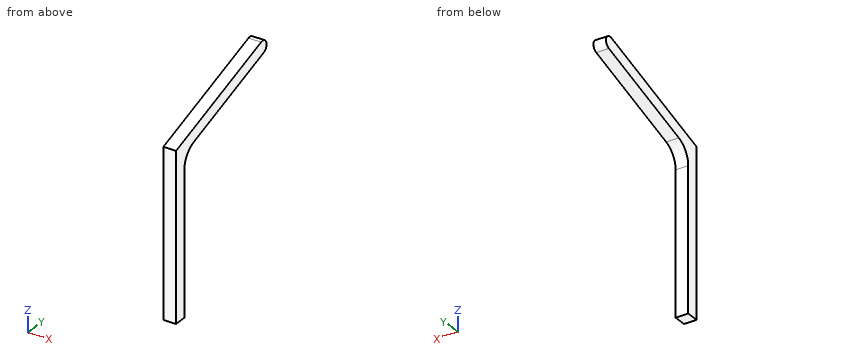
from build123d import *

# Parameters (mm, degrees)
SALIENTE_EXTRUIR1_DEPTH = 6


with BuildPart() as part:
    # Croquis1 → Saliente-Extruir1 (new body)
    with BuildSketch(Plane(origin=(3, 0, 0), x_dir=(0, 0, -1), z_dir=(1, 0, 0))):
        with BuildLine():
            Line((-143.367600492, 342.71356838), (-122.930987198, 281.403728499))
            Line((-122.930987198, 281.403728499), (-43.606431878, 281.403728499))
            Line((-43.606431878, 281.403728499), (-43.606431878, 287.403728499))
            Line((-43.606431878, 287.403728499), (-111.398839678, 287.403728499))
            ThreePointArc((-111.398839678, 287.403728499), (-117.245942524, 289.291306647), (-120.885672658, 294.241450839))
            Line((-120.885672658, 294.241450839), (-137.675500704, 344.610934976))
            ThreePointArc((-137.675500704, 344.610934976), (-141.470233896, 346.508301573), (-143.367600492, 342.71356838))
        make_face()
    extrude(amount=-SALIENTE_EXTRUIR1_DEPTH)


solid = part.part
CAD build for the part. Positions are in the model's coordinates, mm. Round coordinates to 2 decimals unless told otherwise and drop trailing zeros. Write each loop counter-clockwise with the first axis right and the second up, starting at its lowest first coordinate (ties: lowest second). Pieces come first, ordered by that corner, then holes. Notation, with made-up numbers: M 63.25,0.5 L 85.25,0.5 A22 cw 85.25,22.5 Z; hole C -12.5,-18 d8. An arc over 180 degrees is marked long. Put each result on its own line as item: value. Start each with the question number.
1) Pin check, flat tips, straight feed: pin 1 Ø12 at (y, z) = (323.5, 123) entering from -X; pin 2 Ø1.5 at (x, y) = (2, 326) entering from +Z. Stop position of each tip, or through.
2) Saw through at A-A, the plane x = 1.6. Write the cut outline in (y, z).
3) Drill centre lines: probe 1 along Y at (x, z) = (-1.55, 102); probe 2 along Z at (x, y) = (0.55, 327); probe 3 along Z at (x, y) = (-1.4, 330). Where is each one in solid material? Low to high. Write a range as [from, to].
4) Saw through at C-C, the plane y = 296. Write the cut outline in (x, z), and give its area (3 significant figures).
5) Saw through at B-B, the plane z = 59. Write the cut outline in (x, y).
Resolved:
1. pin 1: through
1. pin 2: z = 138.05
2. outline: M 281.4,43.61 L 287.4,43.61 L 287.4,111.4 A10 cw 294.24,120.89 L 344.61,137.68 A3 ccw 342.71,143.37 L 281.4,122.93 Z
3. probe 1: [281.4, 287.4]
3. probe 2: [131.81, 138.13]
3. probe 3: [132.81, 139.13]
4. outline: M -3,121.47 L 3,121.47 L 3,127.8 L -3,127.8 Z
4. area: 37.9 mm²
5. outline: M -3,281.4 L 3,281.4 L 3,287.4 L -3,287.4 Z
